from build123d import *

# Parameters (mm, degrees)
SKETCH4_W       = 0.5
SKETCH4_H       = 3.5
EXTRUDE4_DEPTH  = 2
SKETCH2_W       = 0.5
SKETCH2_H       = 0.25
EXTRUDE_1_DEPTH = 5


with BuildPart() as part:
    # Sketch1 → Revolve1 (revolve)
    with BuildSketch(Plane.XY):
        with BuildLine():
            Line((0, 2.5), (0, -5.5))
            Line((0, -5.5), (0, -6.5))
            Line((0, -6.5), (3, -6.5))
            Line((3, -6.5), (3, -5.5))
            Line((3, -5.5), (2.5, -5.5))
            Line((2.5, -5.5), (2.5, 0))
            ThreePointArc((2.5, 0), (1.767766953, 1.767766953), (0, 2.5))
        make_face()
    revolve(axis=Axis((0, 40.48125, 0), (0, -1, 0)))

    # Sketch4 → Extrude4 (cut)
    with BuildSketch(Plane.XZ.offset(6.5)):
        with Locations((-2.817517664, 0)):
            Rectangle(SKETCH4_W, SKETCH4_H)
    extrude(amount=-EXTRUDE4_DEPTH, mode=Mode.SUBTRACT)

    # Sketch2 → 凸台-拉伸1 (add)
    with BuildSketch(Plane.XZ.offset(6.5)):
        with Locations((1.25, 0)):
            Rectangle(SKETCH2_W, SKETCH2_H)
        with Locations((-1.25, 0)):
            Rectangle(SKETCH2_W, SKETCH2_H)
    extrude(amount=EXTRUDE_1_DEPTH)


solid = part.part
Geometry check sheet. Reference: the model listing, model coordinates, mm. A direction names the side the tool comes from. Give positions to 0.01 mm unless a question says otherwise; leave off trailing zeros. Write each loop counter-clockwise with the first axis right and the second up, starting at its lowest first coordinate (ties: lowest second). Pieces come first, ordered by that corner, then holes.
1) Go/stop test with flat-tipped pins: pin 1 Ø0.6 at (x, y) = (1, -8.5) entering from +Z (3 decimals); pin 2 Ø3 at (x, z) = (1, 0.5) entering from +Y. Record where each tip stops, or that it passes through.
Values follow:
pin 1: stops at z = 0.125
pin 2: stops at y = 2.5
2) Set-up check for faces 1 (the face through (3, -6, 0)), 2 (the face through (2, -5.5, -2)): record each of +Z, -Z, +X, -X, +Y, -Y from which the full face is reachable in a straight line by a thin tool's end or side.
Values follow:
face 1: +Y, -Y
face 2: +Y
3) Thickness scan on line 1 (Y direction, x = -1, z = -2.4); line 2 (Z direction, x = -1.15, y = -7.5) (3 decimals); line 3 (Y direction, x = -0.6, z = 1.3). Record the ranges inside material, lowest first.
Values follow:
line 1: y = -6.5 to -5.5
line 2: z = -0.125 to 0.125
line 3: y = -6.5 to 2.05
4) Cross-section at D-D (y = -3.5). Record the boundary of the cut face in (x, z).
Values follow:
outline: circle Ø5 at (0, 0)
5) Cross-section at C-C (z = -2.05). Record the boundary of the cut face in (x, y), plus the area to 3 significant figures.
Values follow:
outline: (-2.19, -6.5) - (2.19, -6.5) - (2.19, -5.5) - (1.43, -5.5) - (1.43, 0) arc R1.43 ccw to (-1.43, 0) - (-1.43, -5.5) - (-2.19, -5.5) - close
area: 23.3 mm2
6) Cross-section at A-A (y = -9). Record the boundary of the cut face in (x, z) (3 decimals).
Values follow:
outline: (-1.5, -0.125) - (-1, -0.125) - (-1, 0.125) - (-1.5, 0.125) - close; (1, -0.125) - (1.5, -0.125) - (1.5, 0.125) - (1, 0.125) - close
7) Cross-section at B-B (x = 0). Record the boundary of the cut face in (y, z).
Values follow:
outline: (-6.5, -3) - (-5.5, -3) - (-5.5, -2.5) - (0, -2.5) arc R2.5 ccw to (0, 2.5) - (-5.5, 2.5) - (-5.5, 3) - (-6.5, 3) - close
